```python
from build123d import *

# Parameters (mm, degrees)
BOSS_EXTRUDE1_DEPTH = 5
SKETCH2_R           = 1.5
CUT_EXTRUDE1_DEPTH  = 11.07472084


with BuildPart() as part:
    # Sketch1 → Boss-Extrude1 (new body)
    with BuildSketch(Plane(origin=(0, 0, 0), x_dir=(1, 0, 0), z_dir=(0, 1, 0))):
        with BuildLine():
            Line((-3, 0.5), (-3, 2))
            ThreePointArc((-3, 2), (0, 5), (3, 2))
            Line((3, 2), (3, 0.5))
            Line((3, 0.5), (7.5, 0.5))
            Line((7.5, 0.5), (7.5, -0.5))
            Line((7.5, -0.5), (2.449489743, -0.5))
            ThreePointArc((2.449489743, -0.5), (2.487340383, -0.251272405), (2.5, 0))
            Line((2.5, 0), (2.5, 2))
            ThreePointArc((2.5, 2), (0, 4.5), (-2.5, 2))
            Line((-2.5, 2), (-2.5, 0))
            ThreePointArc((-2.5, 0), (-2.487340383, -0.251272405), (-2.449489743, -0.5))
            Line((-2.449489743, -0.5), (-7.5, -0.5))
            Line((-7.5, -0.5), (-7.5, 0.5))
            Line((-7.5, 0.5), (-3, 0.5))
        make_face()
    extrude(amount=BOSS_EXTRUDE1_DEPTH)

    # Sketch2 → Cut-Extrude1 (cut, through all)
    with BuildSketch(Plane(origin=(0, 0, -0.5), x_dir=(-1, 0, 0), z_dir=(0, 0, -1))):
        with Locations((5.008421406, 2.5)):
            Circle(SKETCH2_R)
        with Locations(Location((-5.008421406, 2.5, 0), (0, 0, 180))):
            Circle(SKETCH2_R)
    extrude(amount=-CUT_EXTRUDE1_DEPTH, mode=Mode.SUBTRACT)


solid = part.part
```
Geometry check sheet. Reference: the model listing, model coordinates, mm. A direction names the side the tool comes from. Give positions to 0.01 mm unless a question says otherwise; leave off trailing zeros. Write each loop counter-clockwise with the first axis right and the second up, starting at its lowest first coordinate (ties: lowest second). Pieces come first, ordered by that corner, then holes. Notation, with made-up numbers: (-13, -26) - (7, -26) arc R21 cw to (7, -21) - close; hole circle Ø9 at (-29.5, -12.5). An arc over 180 degrees is marked (long way). Use a Markdown table: item, result.
Q1. Section check D-D, the plane x = 0. Enter the section's corners in (y, z).
Computed:
| item | result |
|---|---|
| outline | (0, -5) - (5, -5) - (5, -4.5) - (0, -4.5) - close |
Q2. Set-up check for faces 1 (the face through (7, 2, -0.5)), 2 (the face through (7.5, 2, 0)), 3 (the face through (-7, 2, -0.5)), 4 (the face through (0.1, 2.5, -4.5)): record each of +Z, -Z, +X, -X, +Y, -Y from which the full face is reachable in a straight line by a thin tool's end or side.
Computed:
| item | result |
|---|---|
| face 1 | -Z, +X, +Y, -Y |
| face 2 | +Z, -Z, +X, +Y, -Y |
| face 3 | -Z, -X, +Y, -Y |
| face 4 | +Y, -Y |
Q3. Draft check along X on faces 5 (the face through (2.5, 2, -1)), 6 (the face through (6, 1, 0.5)), 7 (the face through (-7.5, 2, 0)), 8 (the face through (-6.394, 1.925, -0.007)). Enter one of: pulls with the +X half, pulls with the -X half, needs draft (parallel to the pull), parting line crosses it, or undercut.
Computed:
| item | result |
|---|---|
| face 5 | undercut |
| face 6 | needs draft |
| face 7 | pulls with the -X half |
| face 8 | undercut |
Q4. Section check C-C, the plane x = 5.75. Enter the section's corners in (y, z).
Computed:
| item | result |
|---|---|
| outline | (0, -0.5) - (1.2, -0.5) - (1.2, 0.5) - (0, 0.5) - close; (3.8, -0.5) - (5, -0.5) - (5, 0.5) - (3.8, 0.5) - close |
Q5. Thickness scan on L1, parallel to X at y = 2.9, z = -0.3; L2, parallel to X at y = 2.8, z = -2.85; L3, parallel to X at y = 0.6, z = -3.7. Record the ranges inside material, lowest first. Write a range as [from, to].
Computed:
| item | result |
|---|---|
| L1 | x = [-7.5, -6.45], [-3.56, -2.5], [2.5, 3.56], [6.45, 7.5] |
| L2 | x = [-2.88, -2.35], [2.35, 2.88] |
| L3 | x = [-2.47, -1.83], [1.83, 2.47] |
Q6. Go/stop test with flat-tipped pins: P1, Ø1.6, axis at y = 2, z = -1.5, coming from the +X side; P2, Ø1.8, axis at x = 5.01, y = 2.5, coming from the +Z side; P3, Ø1.2, axis at y = 2, z = -1.5, coming from the -X side; P4, Ø3, axis at x = 2.5, y = 2.5, coming from the -Z side. Record where each tip stops, or that it passes through.
Computed:
| item | result |
|---|---|
| P1 | stops at x = 3 |
| P2 | passes through |
| P3 | stops at x = -3 |
| P4 | stops at z = -4.83 |
Q7. Section check B-B, the plane y = 2.5. Enter the section's corners in (x, z).
Computed:
| item | result |
|---|---|
| outline | (-7.5, -0.5) - (-6.51, -0.5) - (-6.51, 0.5) - (-7.5, 0.5) - close; (-3.51, -0.5) - (-3, -0.5) - (-3, -2) arc R3 ccw to (3, -2) - (3, -0.5) - (3.51, -0.5) - (3.51, 0.5) - (2.45, 0.5) arc R2.5 cw to (2.5, 0) - (2.5, -2) arc R2.5 cw to (-2.5, -2) - (-2.5, 0) arc R2.5 cw to (-2.45, 0.5) - (-3.51, 0.5) - close; (6.51, -0.5) - (7.5, -0.5) - (7.5, 0.5) - (6.51, 0.5) - close |
Q8. Section check A-A, the plane z = -1.1. Enter the section's corners in (x, y), then the cut area to 3 significant figures.
Computed:
| item | result |
|---|---|
| outline | (-3, 0) - (-2.5, 0) - (-2.5, 5) - (-3, 5) - close; (2.5, 0) - (3, 0) - (3, 5) - (2.5, 5) - close |
| area | 5.00 mm² |
